The model under review builds one solid part; all positions refer to its coordinate system, in mm. Coordinates: 2 decimals unless noted, no trailing zeros. Order: outer loops, then holes, each group sorted by start corner. A loop starts at its lowest first (then second) coordinate and runs counter-clockwise, first axis right, second up. Notation, with made-up numbers: (76.5, 8) -> (118.5, 8) arc R15 cw to (118.5, 23) -> close; hole circle Ø4 at (61, 19). An arc over 180 degrees is marked (long way). Use one line per item in the form item = value.
Autodesk Inventor part; units mm, degrees
ref_plane "YZ Plane" through (0, 0, 0) normal (1, 0, 0) x (0, 1, 0)
ref_plane "XZ Plane" through (0, 0, 0) normal (0, 1, 0) x (-1, 0, 0)
ref_plane "XY Plane" through (0, 0, 0) normal (0, 0, 1) x (1, 0, 0)
sketch "Sketch1" plane through (0, 0, 0) normal (0, 0, 1) x (1, 0, 0)
  line L0 (-50, -60.5988) -> (50, -60.5988)
  line L1 (50, -60.5988) -> (50, 60.5988)
  line L2 (50, 60.5988) -> (-50, 60.5988)
  line L3 (-50, 60.5988) -> (-50, -60.5988)
  line L4 (-50, -60.5988) -> (50, 60.5988) construction
  line L5 (50, -60.5988) -> (-50, 60.5988) construction
  point P0 (0, 0)
  dimension "d0" = 100
  dimension "d1" = 121.1976
extrude "Plate1" add sketch "Sketch1" along normal blind 6
fillet "Corner Round1" radius 20 4 edges at (50, -60.5988, 3) (-50, -60.5988, 3) (-50, 60.5988, 3) (50, 60.5988, 3)
sketch "Sketch5" plane through (0, 0, 6) normal (0, 0, 1) x (1, 0, 0)
  line L0 (50, 40.5988) -> (50, -40.5988)
  line L1 (50, 30.5988) -> (-50, 30.5988)
  line L2 (-50, -40.5988) -> (-50, 40.5988)
  line L3 (-30, 60.5988) -> (30, 60.5988)
  point P0 (0, 0)
  dimension "d23" = 30
feature "Fold1" [suppressed]
equation "\"d1\" = Legs_Upper_plate_lenght"
equation "\"d2\" = Thickness"
equation "\"d24\" = BendReliefWidth"
equation "\"d25\" = BendReliefDepth"
equation "\"d26\" = MinimumRemnant"
equation "\"d27\" = TransitionRadius"
equation "\"d29\" = BendRadius"
equation "\"BendReliefWidth\" = Thickness"
equation "\"BendReliefDepth\" = 0.5 * Thickness"
equation "\"CornerReliefSize\" = 4 * Thickness"
equation "\"MinimumRemnant\" = 2 * Thickness"
equation "\"TransitionRadius\" = BendRadius"
equation "\"JacobiRadiusSize\" = BendRadius"
equation "\"GapSize\" = Thickness"
properties part number "PRS 9694 leg plate for filter_D1200 940" material "Stainless Steel"
Item 1: To check wall thickness, follow L1, parallel to Y at x = 36, z = 1.05; L2, parallel to X at y = 46, z = 3.55; L3, parallel to X at y = 44.5, z = 5.6. State the ranges of each line that lie inside material, in increasing order. Write a range as from..to.
Results found:
L1 = -59.68..59.68
L2 = -49.26..49.26
L3 = -49.62..49.62
Item 2: We need section A-A (z = 1.4). Write out the cut boundary in (x, y).
Results found:
outline = (-50, -40.6) arc R20 ccw to (-30, -60.6) -> (30, -60.6) arc R20 ccw to (50, -40.6) -> (50, 40.6) arc R20 ccw to (30, 60.6) -> (-30, 60.6) arc R20 ccw to (-50, 40.6) -> close
Item 3: We need section B-B (x = -42). Write out the cut boundary in (y, z), plus the area to 3 significant figures.
Results found:
outline = (-56.6, 0) -> (56.6, 0) -> (56.6, 6) -> (-56.6, 6) -> close
area = 679 mm²
Item 4: Clearance check with a flat-ended pin moving along its axis: pin 1 (1.5 mm diameter, centred on x = -34.5, z = 4.5, fed in from -Y). State where the tip first meets the part, or that it passes through.
Results found:
pin_1 = -60.24
Item 5: We need section C-C (x = 39). Write out the cut boundary in (y, z), plus the area to 3 significant figures.
Results found:
outline = (-58.46, 0) -> (58.46, 0) -> (58.46, 6) -> (-58.46, 6) -> close
area = 702 mm²
